Here's how the part is built. I have some questions about the finished solid (model axes, mm). A direction names the side the tool comes from. Coordinates: 2 decimals unless noted, no trailing zeros. Loops run counter-clockwise (first coordinate to the right, second up) from the corner with the lowest first, then second, coordinate; pieces in that order, holes last. Notation, with made-up numbers: (74.25, 35.25) -> (121.25, 35.25) arc R30 cw to (121.25, 66.25) -> close; hole circle Ø5 at (44.25, 50). An arc over 180 degrees is marked (long way). Answer as a JSON object with one key per item and string values. Group by question number.
Q1. Thinking about a two-plate mould opening in Y: for faces 1 (the cylindrical face through (5.56, 0.8, -1.05)), 2 (the flat face through (12.7, -1, -1)), 3 (the cylindrical face through (8.926, -37.794, -28.979)), 4 (the conical face through (11.63, 0.07, 0.22)), which applies, released by +Y, released by -Y, zero draft, split by the parting line, or undercut?
Q2. I need wall thicknesses on line 1 (Y direction, x = 9, z = 0) (3 decimals); line 2 (Z direction, x = 6.25, y = 0); line 3 (X direction, y = 4, z = 29). Which ranges of each line are inside material? Lowest first, please.
Q3. I want a section at A-A on x = 2. Write out the boundary of the cut face in (y, z) (3 decimals), then the cut area to 3 significant figures.
Q4. I'm going to push flat-ended pins straight in: pin 1 (1 mm diameter, centred on y = 4.5, z = -26.5, fed in from -X); pin 2 (10 mm diameter, centred on y = -34, z = -35, fed in from +X); pin 3 (6 mm diameter, centred on x = 7.5, y = -29, fed in from +Z). Where does each tip first touch, or does it pass through?
Q5. On a 3-axis mill with a long thin cutter (end or side, diameter ignored), from which of +Z, -Z, +X, -X, +Y, -Y can I reach the whole of each face in a straight line? I mean faces 5 (the cylindrical face through (3.21, -0.69, -3.1)), 6 (the flat face through (0, 1.1, 1.1)). Say none if no direction works.
Q6. I want a section at B-B on x = 8.75. Write out the boundary of the cut face in (y, z) (3 decimals), then the cut area to 3 significant figures.
Autodesk Inventor part; units mm, degrees
ref_plane "YZ Plane" through (0, 0, 0) normal (1, 0, 0) x (0, 1, 0)
ref_plane "XZ Plane" through (0, 0, 0) normal (0, 1, 0) x (-1, 0, 0)
ref_plane "XY Plane" through (0, 0, 0) normal (0, 0, 1) x (1, 0, 0)
sketch "Sketch5" plane through (0, 0, 0) normal (0, 0, 1) x (1, 0, 0)
  line L0 (0, 0) -> (0, 3.175)
  line L1 (0, 3.175) -> (5.715, 3.175)
  line L2 (6.35, 4.191) -> (6.35, 47.625)
  line L3 (6.35, 47.625) -> (12.7, 47.625)
  line L4 (12.7, 47.625) -> (12.7, 0)
  line L5 (12.7, 0) -> (0, 0)
  line L6 (5.715, 3.175) -> (5.715, 4.191)
  line L7 (5.715, 4.191) -> (6.35, 4.191)
  point P0 (9.525, 3.175)
  dimension "d9" = 3.175
  dimension "d10" = 47.625
  dimension "d14" = 6.35
  dimension "d18" = 0.635
  dimension "d19" = 4.191
  dimension "d21" = 5.715
revolve "Revolution1" add sketch "Sketch5" angle 360 about axis through (12.7, 0, 0) along (-1, 0, 0)
fillet "Fillet1" radius 1.27 1 edges at (12.7, -47.625, 0)
chamfer "Chamfer1" distance 0.635 angle 45 1 edges at (0, -3.175, 0)
sketch "Sketch6" plane through (12.7, 0, 0) normal (1, 0, 0) x (0, 0, -1)
  circle A0 centre (0, 0) radius 46.355
  line L0 (-34.925, -19.05) -> (34.925, -19.05)
  line L1 (0, 0) -> (0, -19.05)
  point P0 (0, -43.18)
  dimension "d27" = 43.18
  dimension "d43" = 69.85
  dimension "d44" = 19.05
hole "Hole1" at (12.7, -43.18, 0) direction (-1, 0, 0) diameter 1.524 end through all
sketch "Sketch7" plane through (0, 0, 0) normal (-1, 0, 0) x (0, 0, 1)
  point P0 (0, 0)
hole "Hole2" at (0, 0, 0) direction (1, 0, 0) diameter 2.6416 depth 10.9728 tip angle 118
properties part number "wheel hubcap" material "Aluminum 6061"
Result set:
{
 "1": {"face 1": "undercut", "face 2": "zero draft", "face 3": "split by the parting line", "face 4": "undercut"},
 "2": {"line 1": "y = -47.625 to -43.942, -42.418 to -1.321, 1.321 to 47.625", "line 2": "z = -4.19 to -1.32, 1.32 to 4.19", "line 3": "x = 6.35 to 12.7"},
 "3": {"outline": "circle Ø6.35 at (0, 0); hole circle Ø2.642 at (0, 0)", "area": "26.2 mm²"},
 "4": {"pin 1": "stops at x = 6.35", "pin 2": "stops at x = 12.7", "pin 3": "stops at z = 39.9"},
 "5": {"face 5": "-X", "face 6": "+Z, -Z, -X, +Y, -Y"},
 "6": {"outline": "circle Ø95.25 at (0, 0); hole circle Ø1.524 at (-43.18, 0); hole circle Ø2.642 at (0, 0)", "area": "7,120 mm²"}
}
